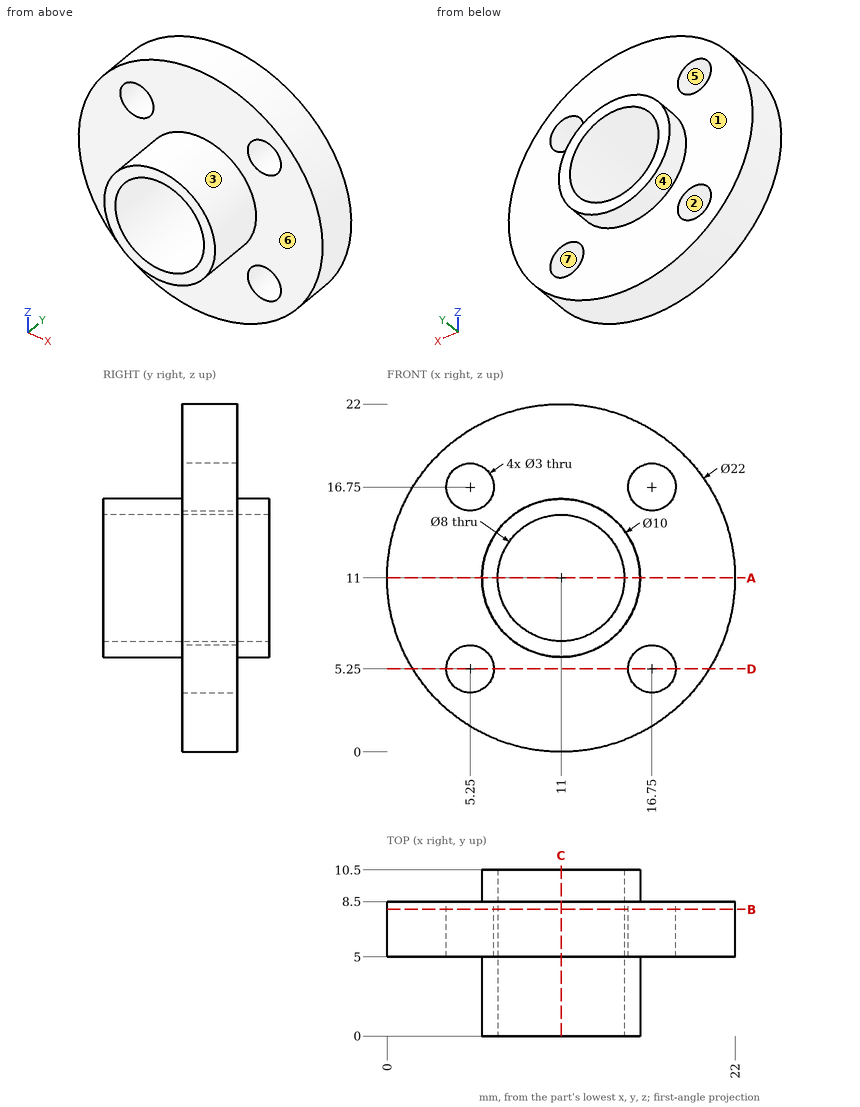
Drawing for the job (mm, zero at the part's lowest x, y, z). A direction names the side the tool comes from. Give positions to 0.01 mm unless a question says otherwise; leave off trailing zeros. Loops run counter-clockwise (first coordinate to the right, second up) from the corner with the lowest first, then second, coordinate; pieces in that order, holes last. Notation, with made-up numbers: (-12, -19) - (-6, -19) arc R16 ccw to (-6, -4) - close; hole circle Ø1 at (59.5, 18). An arc over 180 degrees is marked (long way). Write item = value, one per line. Start each with the question number.
1) Band-saw the part on D-D on z = 5.25. Give the cut face in (x, y).
2) Pull direction X, two halves, no side cores. Call the marked faces 4, 5, 6 and 7: +X half, -X half, draft (parallel to the pull), parting line (faces both ways), or undercut.
3) Tool access for the marked faces 1, 2 and 3: list every direction of +Z, -Z, +X, -X, +Y, -Y with a clear straight run to the whole face (end or side of a thin tool).
4) Probe probe 1 along X at (y, z) = (7.4, 16.75); probe 2 along X at (y, z) = (3.75, 11); probe 3 along Y at (x, z) = (4.5, 12.5). List the from-to ranges inside material, lowest first. Write a range as from..to.
5) Drop flat-ended pins along their axis: pin 1 Ø5 at (x, y) = (19.5, 6.5) entering from -Z; pin 2 Ø1.8 at (x, z) = (5.25, 16.75) entering from -Y; pin 3 Ø3.5 at (x, z) = (5.25, 5.25) entering from +Y; pin 4 Ø8 at (x, z) = (4, 7) entering from +Y. Give the stop position or say it passes through.
6) Band-saw the part on C-C on x = 11. Give the cut face in (y, z).
7) Band-saw the part on B-B on y = 8. Give the cut face in (x, z), plus the area to 3 significant figures.
8) Band-saw the part on A-A on z = 11. Give the cut face in (x, y), plus the area to 3 significant figures.
Final values:
q1.outline = (1.62, 5) - (3.75, 5) - (3.75, 8.5) - (1.62, 8.5) - close; (6.75, 5) - (15.25, 5) - (15.25, 8.5) - (6.75, 8.5) - close; (18.25, 5) - (20.38, 5) - (20.38, 8.5) - (18.25, 8.5) - close
q2.face_4 = parting line
q2.face_5 = undercut
q2.face_6 = draft
q2.face_7 = undercut
q3.face_1 = +Y
q3.face_2 = +Y, -Y
q3.face_3 = -Y
q4.probe_1 = 1.62..3.75, 6.75..15.25, 18.25..20.38
q4.probe_2 = 6..7, 15..16
q4.probe_3 = 5..8.5
q5.pin_1 = 1.78
q5.pin_2 = through
q5.pin_3 = 8.5
q5.pin_4 = 10.5
q6.outline = (0, 6) - (5, 6) - (5, 0) - (8.5, 0) - (8.5, 6) - (10.5, 6) - (10.5, 7) - (0, 7) - close; (0, 15) - (10.5, 15) - (10.5, 16) - (8.5, 16) - (8.5, 22) - (5, 22) - (5, 16) - (0, 16) - close
q7.outline = circle Ø22 at (11, 11); hole circle Ø3 at (5.25, 5.25); hole circle Ø3 at (5.25, 16.75); hole circle Ø8 at (11, 11); hole circle Ø3 at (16.75, 5.25); hole circle Ø3 at (16.75, 16.75)
q7.area = 302 mm²
q8.outline = (0, 5) - (6, 5) - (6, 0) - (7, 0) - (7, 10.5) - (6, 10.5) - (6, 8.5) - (0, 8.5) - close; (15, 0) - (16, 0) - (16, 5) - (22, 5) - (22, 8.5) - (16, 8.5) - (16, 10.5) - (15, 10.5) - close
q8.area = 63.0 mm²
